Build history of the part. All positions in model axes, mm. Give positions to 0.01 mm unless a question says otherwise; leave off trailing zeros. Write each loop counter-clockwise with the first axis right and the second up, starting at its lowest first coordinate (ties: lowest second). Pieces come first, ordered by that corner, then holes. Notation, with made-up numbers: M -1.5,-8.5 L 15.5,-8.5 A17 ccw 15.5,17.5 Z; hole C 58,-22 d10. An arc over 180 degrees is marked long. Return JSON: item names as keys, results as strings. Group by question number.
Q1. Band-saw the part on B-B, the plane y = 0. Give the cut face in (x, z) (1 decimal), then the cut area to 3 significant figures.
Q2. Flat gauge pin, fed straight in: pin 1 Ø2.5 at (x, y) = (0, 28.575) entering from +Z. Where does the tip first touch, or does it go through?
Q3. Band-saw the part on A-A, the plane x = 0. Give the cut face in (y, z) (1 decimal), then the cut area to 3 significant figures.
Q4. Wall check: probe 1 along Y at (x, z) = (38.1, 2.05); probe 2 along Y at (x, z) = (1, 2.8). Give the ranges that are in metal, low to high.
Q5. Pull direction Y, two halves, no side cores. Call faces 1 (the cylindrical face through (-0.344, 27.025, 1.565)), 2 (the flat face through (19, 15, 0)), 3 (the flat face through (19, -17.462, 2)), 4 (the flat face through (19, 46.038, 2)): +Y half, -Y half, draft (parallel to the pull), parting line (faces both ways), or undercut.
from build123d import *

# Parameters (mm, degrees)
SKETCH1_W           = 69.85
SKETCH1_H           = 63.5
SKETCH1_R           = 1.5875
BOSS_EXTRUDE1_DEPTH = 3.175


with BuildPart() as part:
    # Sketch1 → Boss-Extrude1 (new body)
    with BuildSketch(Plane.XY):
        with Locations((19.05, 14.2875)):
            Rectangle(SKETCH1_W, SKETCH1_H)
        with Locations((0, 28.575)):
            Circle(SKETCH1_R, mode=Mode.SUBTRACT)
        with Locations((38.1, 28.575)):
            Circle(SKETCH1_R, mode=Mode.SUBTRACT)
        with Locations((38.1, 0)):
            Circle(SKETCH1_R, mode=Mode.SUBTRACT)
        Circle(SKETCH1_R, mode=Mode.SUBTRACT)
    extrude(amount=BOSS_EXTRUDE1_DEPTH)


solid = part.part
From the geometry:
{
 "1": {"outline": "M -15.9,0 L -1.6,0 L -1.6,3.2 L -15.9,3.2 Z; M 1.6,0 L 36.5,0 L 36.5,3.2 L 1.6,3.2 Z; M 39.7,0 L 54,0 L 54,3.2 L 39.7,3.2 Z", "area": "202 mm^2"},
 "2": {"pin 1": "passes through"},
 "3": {"outline": "M -17.5,0 L -1.6,0 L -1.6,3.2 L -17.5,3.2 Z; M 1.6,0 L 27,0 L 27,3.2 L 1.6,3.2 Z; M 30.2,0 L 46,0 L 46,3.2 L 30.2,3.2 Z", "area": "181 mm^2"},
 "4": {"probe 1": "y = -17.46 to -1.59, 1.59 to 26.99, 30.16 to 46.04", "probe 2": "y = -17.46 to -1.23, 1.23 to 27.34, 29.81 to 46.04"},
 "5": {"face 1": "undercut", "face 2": "draft", "face 3": "-Y half", "face 4": "+Y half"}
}
